Autodesk Inventor part; units mm, degrees
ref_plane "YZ Plane" through (0, 0, 0) normal (1, 0, 0) x (0, 1, 0)
ref_plane "XZ Plane" through (0, 0, 0) normal (0, 1, 0) x (-1, 0, 0)
ref_plane "XY Plane" through (0, 0, 0) normal (0, 0, 1) x (1, 0, 0)
sketch "Sketch1" plane through (0, 0, 0) normal (0, 0, 1) x (1, 0, 0)
  line L0 (0, 0) -> (167, 0)
  line L1 (167, 0) -> (167, 10)
  line L2 (167, 10) -> (0, 10)
  line L3 (0, 10) -> (0, 0)
  circle A0 centre (59.5, 5) radius 1.6
  circle A1 centre (101.5, 5) radius 1.6
  circle A2 centre (162, 5) radius 1.6
  circle A3 centre (149.5, 5) radius 1.6
  circle A4 centre (15, 5) radius 1.6
  circle A5 centre (5, 5) radius 1.6
  dimension "d1" = 10
  dimension "d2" = 90
  dimension "d4" = 3.2
  dimension "d6" = 3.2
  dimension "d7" = 3.2
  dimension "d8" = 42
  dimension "d9" = 60.5
  dimension "d26" = 3.2
  dimension "d27" = 48
  dimension "d28" = 3.2
  dimension "d29" = 44.5
  dimension "d32" = 15
  dimension "d33" = 5
  dimension "d61" = 3.2
  dimension "d62" = 10
  dimension "d63" = 12.5
ref_plane "Work Plane2" through (0, 0, 0) normal (0, -1, 0) x (1, 0, 0)
sketch "Sketch2" plane through (0, 0, 0) normal (0, -1, 0) x (1, 0, 0)
  circle A0 centre (54.5, 7) radius 1.6
  circle A1 centre (124.5, 7) radius 1.6
  circle A2 centre (89.5, 7) radius 1.6
  point P0 (0, 0)
  dimension "d13" = 3.2
  dimension "d15" = 3.2
  dimension "d16" = 70
  dimension "d17" = 3.2
  dimension "d18" = 35
  dimension "d64" = 54.5
  dimension "d65" = 35
ref_plane "Work Plane1" through (0, 0, 11) normal (0, 0, 1) x (1, 0, 0)
extrude "klocek" add sketch "Sketch1" along normal blind 11
ref_plane "Work Plane3" through (0, 0, 0) normal (0, -1, 0) x (1, 0, 0)
extrude "prowadzenie osi" cut sketch "Sketch2" against normal up to next
ref_plane "Work Plane4" through (0, 0, 0) normal (0, -1, 0) x (1, 0, 0)
sketch "Sketch7" plane through (0, 0, 0) normal (0, -1, 0) x (1, 0, 0)
  line L0 (0, 11) -> (0, 0)
  line L1 (0, 11) -> (167, 11)
  line L2 (0, 11) -> (40, 11)
  line L3 (40, 11) -> (0, 0)
  point P0 (0, -1.8333)
  dimension "d86" = 11
  dimension "d87" = 40
sketch "Sketch8" plane through (0, 0, 0) normal (0, -1, 0) x (1, 0, 0)
  line L0 (167, 0) -> (167, 11)
  line L1 (167, 11) -> (167, 3)
  line L2 (167, 11) -> (0, 11)
  line L3 (167, 11) -> (137, 11)
  line L4 (137, 11) -> (167, 3)
  point P0 (0, 0)
  point P1 (40.8333, 11)
  dimension "d80" = 8
  dimension "d81" = 30
extrude "przedni skos" cut sketch "Sketch7" against normal up to next
extrude "tylni skos" cut sketch "Sketch8" against normal up to next
ref_plane "Work Plane7" through (0, 0, 11) normal (0, 0, 1) x (1, 0, 0)
sketch "Sketch5" plane through (0, 0, 11) normal (0, 0, 1) x (1, 0, 0)
  line L0 (62.9064, 5) -> (61.2032, 2.05)
  line L1 (61.2032, 2.05) -> (57.7968, 2.05)
  line L2 (57.7968, 2.05) -> (56.0936, 5)
  line L3 (56.0936, 5) -> (57.7968, 7.95)
  line L4 (57.7968, 7.95) -> (61.2032, 7.95)
  line L5 (61.2032, 7.95) -> (62.9064, 5)
  circle A0 centre (101.5, 5) radius 1.6
  line L6 (98.0936, 5) -> (99.7968, 7.95)
  line L7 (99.7968, 7.95) -> (103.2032, 7.95)
  line L8 (103.2032, 7.95) -> (104.9064, 5)
  line L9 (104.9064, 5) -> (103.2032, 2.05)
  line L10 (103.2032, 2.05) -> (99.7968, 2.05)
  line L11 (99.7968, 2.05) -> (98.0936, 5)
  point P0 (59.5, 5)
  point P1 (119.5, 5)
  dimension "d45" = 5.9
  dimension "d98" = 5.9
extrude "hex insert middle" cut sketch "Sketch5" against normal blind 3
ref_plane "Work Plane6" through (0, 0, 11) normal (0, 0, 1) x (1, 0, 0)
sketch "Sketch9" plane through (0, 0, 11) normal (0, 0, 1) x (1, 0, 0)
  circle A0 centre (149.5, 5) radius 1.6
  line L0 (152.9064, 5) -> (151.2032, 2.05)
  line L1 (151.2032, 2.05) -> (147.7968, 2.05)
  line L2 (147.7968, 2.05) -> (146.0936, 5)
  line L3 (146.0936, 5) -> (147.7968, 7.95)
  line L4 (147.7968, 7.95) -> (151.2032, 7.95)
  line L5 (151.2032, 7.95) -> (152.9064, 5)
  point P0 (0, 0)
  point P1 (153, 5)
  dimension "d99" = 5.9
extrude "hex insert rear 1" cut sketch "Sketch9" against normal blind 6
ref_plane "Work Plane5" through (0, 0, 11) normal (0, 0, 1) x (1, 0, 0)
sketch "Sketch10" plane through (0, 0, 11) normal (0, 0, 1) x (1, 0, 0)
  line L0 (160.2968, 7.95) -> (163.7032, 7.95)
  line L1 (163.7032, 7.95) -> (165.4064, 5)
  line L2 (165.4064, 5) -> (163.7032, 2.05)
  line L3 (163.7032, 2.05) -> (160.2968, 2.05)
  line L4 (160.2968, 2.05) -> (158.5936, 5)
  line L5 (158.5936, 5) -> (160.2968, 7.95)
  point P0 (0, 0)
  point P1 (162, 5)
  point P2 (162, 5)
  dimension "d72" = 5.9
extrude "hex insert rear 2" cut sketch "Sketch10" against normal blind 8.5
sketch "Sketch13" plane through (0, 0, 11) normal (0, 0, 1) x (1, 0, 0)
  circle A0 centre (5, 5) radius 1.6
  line L0 (8.4064, 5) -> (6.7032, 2.05)
  line L1 (6.7032, 2.05) -> (3.2968, 2.05)
  line L2 (3.2968, 2.05) -> (1.5936, 5)
  line L3 (1.5936, 5) -> (3.2968, 7.95)
  line L4 (3.2968, 7.95) -> (6.7032, 7.95)
  line L5 (6.7032, 7.95) -> (8.4064, 5)
  point P0 (0, 0)
  dimension "d90" = 5.9
extrude "hex insert front 1" cut sketch "Sketch13" against normal through all
sketch "Sketch16" plane through (0, 0, 11) normal (0, 0, 1) x (1, 0, 0)
  circle A0 centre (15, 5) radius 1.6
  line L0 (18.4064, 5) -> (16.7032, 2.05)
  line L1 (16.7032, 2.05) -> (13.2968, 2.05)
  line L2 (13.2968, 2.05) -> (11.5936, 5)
  line L3 (11.5936, 5) -> (13.2968, 7.95)
  line L4 (13.2968, 7.95) -> (16.7032, 7.95)
  line L5 (16.7032, 7.95) -> (18.4064, 5)
  point P0 (0, 0)
  dimension "d93" = 5.9
extrude "hex insert front 2" cut sketch "Sketch16" against normal blind 9
sketch "Sketch17" plane through (0, 0, 0) normal (0, 0, -1) x (-1, 0, 0)
  line L0 (0, 10) -> (0, 0)
  line L1 (0, 0) -> (-3.2968, 0)
  line L2 (-3.2968, 0) -> (-3.2968, 10.0042)
  line L3 (-3.2968, 10.0042) -> (0, 10.0042)
  line L4 (0, 10.0042) -> (0, 0)
extrude "Extrusion20" cut sketch "Sketch17" against normal up to next
properties part number "wheel_support_extra_short"
Could you check a few things on this model? Use its own coordinates, in mm. A direction names the side the tool comes from. Coordinates: 2 decimals unless noted, no trailing zeros. Loops run counter-clockwise (first coordinate to the right, second up) from the corner with the lowest first, then second, coordinate; pieces in that order, holes last. Notation, with made-up numbers: (-30, -1.5) -> (26, -1.5) arc R9 cw to (26, 5.5) -> close; hole circle Ø8 at (-19.5, 39). An arc over 180 degrees is marked (long way). Answer in a Markdown table with one row per item.
(1) For faces 1 (the face through (15, 2.05, 3)), 2 (the face through (167, 5, 1)), which set-ups out of +Z, -Z, +X, -X, +Y, -Y let a thin tool reach every point of the face, with its end or its side?
Results found:
| item | result |
|---|---|
| face 1 | +Z |
| face 2 | +Z, -Z, +X, +Y, -Y |
(2) Imagine slicing it at B-B (x = 15). List the corners of the cut face in (y, z) for me (3 decimals), plus the area to 3 significant figures.
Results found:
| item | result |
|---|---|
| outline | (0, 0) -> (3.4, 0) -> (3.4, 2) -> (2.05, 2) -> (2.05, 4.125) -> (0, 4.125) -> close; (6.6, 0) -> (10, 0) -> (10, 4.125) -> (7.95, 4.125) -> (7.95, 2) -> (6.6, 2) -> close |
| area | 22.3 mm^2 |
(3) Thinking about a two-plate mould opening in Y: for faces 3 (the face through (88, 5, 11)), 4 (the face through (84, 0, 5)), 5 (the face through (61.026, 4.519, 3.944)), which applies, released by +Y, released by -Y, zero draft, split by the parting line, or undercut?
Results found:
| item | result |
|---|---|
| face 3 | zero draft |
| face 4 | released by -Y |
| face 5 | undercut |
(4) Imagine slicing it at A-A (x = 54.5). List the corners of the cut face in (y, z) for me, plus the area to 3 significant figures.
Results found:
| item | result |
|---|---|
| outline | (0, 0) -> (10, 0) -> (10, 5.4) -> (0, 5.4) -> close; (0, 8.6) -> (10, 8.6) -> (10, 11) -> (0, 11) -> close |
| area | 78.0 mm^2 |
(5) If I drill on probe 1 along Z at (x, y) = (124.5, 6); probe 2 along Y at (x, z) = (59.5, 6); probe 3 along Z at (x, y) = (143, 3), over which ranges is the centre line in solid material (lowest first)?
Results found:
| item | result |
|---|---|
| probe 1 | z = 0 to 5.4, 8.6 to 11 |
| probe 2 | y = 0 to 3.4, 6.6 to 10 |
| probe 3 | z = 0 to 9.4 |
(6) Will these pins go through, and if not, where does the flat tip stop? pin 1 Ø3.5 at (x, y) = (59.5, 5) entering from +Z; pin 2 Ø1.8 at (x, y) = (15, 4) entering from +Z; pin 3 Ø3 at (x, y) = (162, 4.5) entering from +Z.
Results found:
| item | result |
|---|---|
| pin 1 | stops at z = 8 |
| pin 2 | stops at z = 2 |
| pin 3 | stops at z = 2.5 |
